Geometry: final body of the model. Coordinates: model frame, mm. A direction names the side the tool comes from. Give positions to 0.01 mm unless a question says otherwise; leave off trailing zeros. Write each loop counter-clockwise with the first axis right and the second up, starting at its lowest first coordinate (ties: lowest second). Pieces come first, ordered by that corner, then holes. Notation, with made-up numbers: (-38, 52) -> (-14, 52) arc R24 ccw to (-14, 78) -> close; hole circle Ø8 at (43, 24). An arc over 180 degrees is marked (long way). Use CSV: the item, a comma, the result in double quotes. Start each with the question number.
1) Section D-D (x = 37.5). Output: boundary loops of the cut face in (y, z), plus the area to 3 significant figures.
2) Material intervals for line 1 (Z direction, x = 37, y = 131); line 2 (Y direction, x = 28, z = 15.5); line 3 (Y direction, x = 93.5, z = 23), sorted ascending. Write a range as [from, to].
3) Set-up query: faces 1 (the face through (3.759, 36.435, 20.14)), 2 (the face through (80, 50, 20)), 3 (the face through (17.8, 82.5, 20.1)), 4 (the face through (85.742, 134.964, 5.07)), 5 (the face through (49, 76, 0)). Return all of +Z, -Z, +X, -X, +Y, -Y with unobstructed straight access to the full face (end or side cutting, diameter ignored); none if empty.
4) Section A-A (y = 51). Output: boundary loops of the cut face in (x, z).
5) Draft query along X for faces 6 (the face through (49, 33, 30)), 7 (the face through (15.036, 135.742, 5.07)), 8 (the face through (94.82, 69.86, 20.14)), 9 (the face through (38.094, 67.262, 19.86)). Return one class per face: pulls with the +X half, pulls with the -X half, needs draft (parallel to the pull), parting line crosses it, or undercut.
6) Contact query for flat-ended pins moving along their axis: P1, Ø3, axis at y = 78, z = 20.5, coming from the +X side; P2, Ø2, axis at y = 58, z = 19.5, coming from the -X side; P3, Ø3, axis at x = 67.5, y = 96, coming from the +Z side; P4, Ø2, axis at y = 28, z = 13, coming from the +X side. Output: stop coordinate, or through.
7) Section C-C (x = 21.5). Output: boundary loops of the cut face in (y, z), plus the area to 3 significant figures.
Autodesk Inventor part; units mm, degrees
ref_plane "YZ Plane" through (0, 0, 0) normal (1, 0, 0) x (0, 1, 0)
ref_plane "XZ Plane" through (0, 0, 0) normal (0, 1, 0) x (-1, 0, 0)
ref_plane "XY Plane" through (0, 0, 0) normal (0, 0, 1) x (1, 0, 0)
sketch "Sketch9" plane through (0, 0, 0) normal (0, 0, 1) x (1, 0, 0)
  line L0 (0, 0) -> (100, 0)
  line L1 (100, 0) -> (100, 150)
  line L2 (100, 150) -> (0, 150)
  line L3 (0, 150) -> (0, 0)
  dimension "d68" = 100
  dimension "d69" = 150
extrude "Extrusion8" add sketch "Sketch9" along normal blind 10
sketch "Sketch10" plane through (0, 0, 10) normal (0, 0, 1) x (1, 0, 0)
  line L0 (0, 150) -> (0, 0)
  line L1 (0, 0) -> (100, 0)
  line L2 (100, 0) -> (100, 20)
  line L3 (100, 20) -> (0, 20)
  line L4 (0, 20) -> (0, 0)
  line L5 (50, 20) -> (0, 70)
  line L6 (0, 70) -> (17.6777, 87.6777)
  line L7 (17.6777, 87.6777) -> (67.6777, 37.6777)
  line L8 (67.6777, 37.6777) -> (50, 20)
  line L9 (50, 20) -> (120.7107, 20) construction
  line L10 (50, 20) -> (100, 70)
  line L11 (100, 70) -> (82.3223, 87.6777)
  line L12 (82.3223, 87.6777) -> (32.3223, 37.6777)
  line L13 (32.3223, 37.6777) -> (50, 20)
  line L14 (50, 20) -> (120.7107, 20) construction
  line L15 (0, 20) -> (100, 20)
  line L16 (100, 20) -> (100, 40)
  line L17 (100, 40) -> (0, 40)
  line L18 (0, 40) -> (0, 20)
  point P0 (70, 40)
  point P1 (65.3553, 40)
  point P2 (50, 55.3553)
  point P3 (30, 40)
  dimension "d72" = 100
  dimension "d73" = 20
  dimension "d74" = 135
  dimension "d75" = 25
  dimension "d76" = 45
  dimension "d77" = 25
  dimension "d78" = 20
extrude "Extrusion9" add sketch "Sketch10" along normal blind 20 contours L6 L7 L12 L17 L5 | L17 L5 L3 L0 | L17 L12 L5 | L3 L2 L1 L0 | L12 L17 L7 L8 L5 | L12 L7 L17 | L12 L11 L10 L17 L7 | L8 L10 L17 L16 L3 | L17 L10 L7
fillet "Fillet8" radius 50 2 edges at (0, 150, 5) (100, 150, 5)
fillet "Fillet9" radius 12.5 6 edges at (17.6777, 87.6777, 20) (0, 70, 20) (82.3223, 87.6777, 20) (100, 70, 20) (0, 40, 20) (100, 40, 20)
properties part number "Marker Holder 90 deg"
Answers follow:
1,outline,"(0, 0) -> (148.41, 0) -> (148.41, 10) -> (67.86, 10) -> (67.86, 30) -> (0, 30) -> close"
1,area,"2,840 mm^2"
2,line 1,"z = [0, 10]"
2,line 2,"y = [0, 40], [42, 77.36]"
2,line 3,"y = [0, 38.47], [64.4, 75.6]"
3,face 1,"+Z, -X"
3,face 2,"+Z, +X"
3,face 3,"+Z, +Y"
3,face 4,"+Z, -Z, +X, +Y"
3,face 5,"-Z, +X, -X, +Y, -Y"
4,outline,"(0, 0) -> (100, 0) -> (100, 10) -> (81, 10) -> (81, 30) -> (19, 30) -> (19, 10) -> (0, 10) -> close"
5,face 6,"needs draft"
5,face 7,"pulls with the -X half"
5,face 8,"pulls with the +X half"
5,face 9,"undercut"
6,P1,"stops at x = 93"
6,P2,"stops at x = 11"
6,P3,"stops at z = 10"
6,P4,"stops at x = 100"
7,outline,"(0, 0) -> (141.08, 0) -> (141.08, 10) -> (81.9, 10) -> (81.9, 30) -> (48.5, 30) -> (48.5, 10) -> (40, 10) -> (40, 30) -> (0, 30) -> close"
7,area,"2,880 mm^2"
